Could you check a few things on this drawing? It's one solid part, dimensions in mm from its lowest x, y, z. A direction names the side the tool comes from. Give positions to 0.01 mm unless a question says otherwise; leave off trailing zeros. Order: outer loops, then holes, each group sorted by start corner. A loop starts at its lowest first (then second) coordinate and runs counter-clockwise, first axis right, second up. Notation, with made-up numbers: (21, -15) -> (71, -15) arc R16 ccw to (71, 6) -> close; hole circle Ø3 at (44, 3.25). An arc over 180 degrees is marked (long way). Answer as CSV lines item,"result".
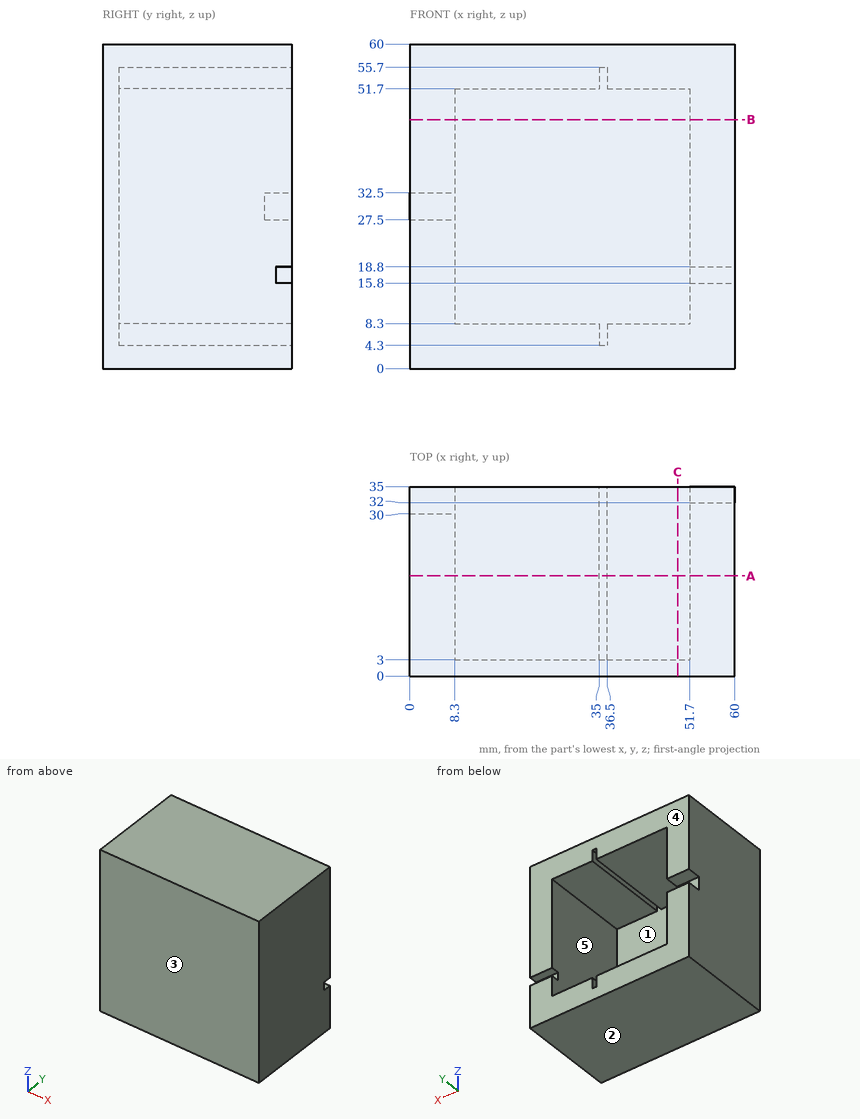
Item 1: Imagine slicing it at C-C, the plane x = 49.5. Please give me the cut outline in (y, z), then the cut area to 3 significant figures.
Numbers:
outline,"(0, 0) -> (35, 0) -> (35, 8.3) -> (3, 8.3) -> (3, 51.7) -> (35, 51.7) -> (35, 60) -> (0, 60) -> close"
area,"711 mm²"
Item 2: Please list where these lines run through material, in increasing order: line 1 along X through (y, z) = (7, 51); line 2 along X through (y, z) = (19.5, 53).
Numbers:
line 1,"x = 0 to 8.3, 51.7 to 60"
line 2,"x = 0 to 35, 36.5 to 60"
Item 3: For pin 1 (1.5 mm diameter, centred on x = 57.5, z = 17.5, fed in from +Y); pin 2 (13 mm diameter, centred on x = 25, z = 23.5, fed in from +Y), each with a flat end and sliding along its axis, tell me the tip position at first contact or that it passes through.
Numbers:
pin 1,"stops at y = 32"
pin 2,"stops at y = 3"
Item 4: Imagine slicing it at A-A, the plane y = 18.5. Please give me the cut outline in (x, z), then the cut area to 3 significant figures.
Numbers:
outline,"(0, 0) -> (60, 0) -> (60, 60) -> (0, 60) -> close; hole (8.3, 8.3) -> (35, 8.3) -> (35, 4.3) -> (36.5, 4.3) -> (36.5, 8.3) -> (51.7, 8.3) -> (51.7, 51.7) -> (36.5, 51.7) -> (36.5, 55.7) -> (35, 55.7) -> (35, 51.7) -> (8.3, 51.7) -> close"
area,"1,700 mm²"
Item 5: Imagine slicing it at B-B, the plane z = 46. Please give me the cut outline in (x, y), then the cut area to 3 significant figures.
Numbers:
outline,"(0, 0) -> (60, 0) -> (60, 35) -> (51.7, 35) -> (51.7, 3) -> (8.3, 3) -> (8.3, 35) -> (0, 35) -> close"
area,"711 mm²"
Item 6: We'd pull the mould along Z, two halves only. Please class the marked faces 1, 2 and 3: released by +Z, released by -Z, zero draft, split by the parting line, or undercut.
Numbers:
face 1,"undercut"
face 2,"released by -Z"
face 3,"zero draft"
Item 7: For the marked faces 4 and 5, which set-ups out of +Z, -Z, +X, -X, +Y, -Y let a thin tool reach every point of the face, with its end or its side?
Numbers:
face 4,"+Z, -Z, +X, -X, +Y"
face 5,"+Y"
